Part model, mm, in its own coordinate system. Round coordinates to 2 decimals unless told otherwise and drop trailing zeros. Loops run counter-clockwise (first coordinate to the right, second up) from the corner with the lowest first, then second, coordinate; pieces in that order, holes last.
from build123d import *

# Parameters (mm, degrees)
F1_DEPTH = 5
F2_R     = 5
F3_SIZE  = 1


with BuildPart() as f1:
    # F0 (on Top) → F1 (new body)
    with BuildSketch(Plane.XY):
        with BuildLine():
            ThreePointArc((4.0489926269, -57.0063869992), (41.8181923846, -38.9533218826), (57.15, 0))
            ThreePointArc((57.15, 0), (55.6922778867, 12.8254701198), (51.3934756327, 24.996663025))
            ThreePointArc((51.3934756327, 24.996663025), (49.4933518263, 28.575), (47.3444830059, 32.0097239742))
            ThreePointArc((47.3444830059, 32.0097239742), (0, 57.15), (-47.3444830059, 32.0097239742))
            ThreePointArc((-47.3444830059, 32.0097239742), (-49.4933518263, 28.575), (-51.3934756327, 24.996663025))
            ThreePointArc((-51.3934756327, 24.996663025), (-49.4933518263, -28.575), (-4.0489926269, -57.0063869992))
            ThreePointArc((-4.0489926269, -57.0063869992), (0, -57.15), (4.0489926269, -57.0063869992))
        make_face()
        with BuildLine():
            ThreePointArc((47.3444830059, 32.0097239742), (49.4933518263, 28.575), (51.3934756327, 24.996663025))
            ThreePointArc((51.3934756327, 24.996663025), (65.9478344982, 38.075), (47.3444830059, 32.0097239742))
        make_face()
        with BuildLine():
            ThreePointArc((-51.3934756327, 24.996663025), (-49.4933518263, 28.575), (-47.3444830059, 32.0097239742))
            ThreePointArc((-47.3444830059, 32.0097239742), (-65.9478344982, 38.075), (-51.3934756327, 24.996663025))
        make_face()
        with BuildLine():
            ThreePointArc((-4.0489926269, -57.0063869992), (0, -76.15), (4.0489926269, -57.0063869992))
            ThreePointArc((4.0489926269, -57.0063869992), (0, -57.15), (-4.0489926269, -57.0063869992))
        make_face()
    extrude(amount=F1_DEPTH)

    # F2
    f2_edges = [f1.edges().sort_by_distance(p)[0] for p in [
        (51.393476, 24.996663, 2.5),
        (-4.048993, -57.006387, 2.5),
        (-47.344483, 32.009724, 2.5),
        (47.344483, 32.009724, 2.5),
        (-51.393476, 24.996663, 2.5),
        (4.048993, -57.006387, 2.5),
    ]]
    fillet(f2_edges, radius=F2_R)

    # F3
    f3_edges = [f1.edges().sort_by_distance(p)[0] for p in [
        (0, 57.15, 5),
        (45.702262, 37.347671, 5),
        (-45.702262, 37.347671, 5),
        (65.947834, 38.075, 5),
        (-65.947834, 38.075, 5),
        (55.195163, 20.905484, 5),
        (-55.195163, 20.905484, 5),
        (49.493352, -28.575, 5),
        (-49.493352, -28.575, 5),
        (9.492901, -58.253155, 5),
        (-9.492901, -58.253155, 5),
        (0, -76.15, 5),
    ]]
    chamfer(f3_edges, length=F3_SIZE)


solid = f1.part
1) Wall check: line 1 along X through (y, z) = (0, 1.35); line 2 along X through (y, z) = (-9.5, 0.6); line 3 along Y through (x, z) = (46, 4.3). Give the ranges that are in metal, low to high.
Values:
line 1: x = -57.15 to 57.15
line 2: x = -56.35 to 56.35
line 3: y = -33.41 to 37.07
2) Mould opens along X. For faces 1 (the face through (-0.251, -75.32, 4.826)), 2 (the face through (-1, 6, 5)), 3 (the face through (66.1, 37.8, 2)) say: released by +X, released by -X, zero draft, split by the parting line, or undercut.
Values:
face 1: split by the parting line
face 2: zero draft
face 3: undercut
3) Drop flat-ended pins along their axis: pin 1 Ø1.5 at (y, z) = (-14, 1.5) entering from +X; pin 2 Ø1.5 at (y, z) = (-46.5, 3) entering from +X. Give the stop position or say it passes through.
Values:
pin 1: stops at x = 55.59
pin 2: stops at x = 34.25
4) Slice it at A-A, the plane y = -66.15. Give the cut face in (x, z), then the cut area to 3 significant figures.
Values:
outline: (-10, 0) - (10, 0) - (10, 4) - (9, 5) - (-9, 5) - (-10, 4) - close
area: 99.0 mm2
